CAD build for the part. Positions are in the model's coordinates, mm. A direction names the side the tool comes from. Round coordinates to 2 decimals unless told otherwise and drop trailing zeros. Loops run counter-clockwise (first coordinate to the right, second up) from the corner with the lowest first, then second, coordinate; pieces in that order, holes last. Notation, with made-up numbers: (-20, -25) - (-16, -25) arc R34 cw to (-16, 7) - close; hole circle Ø9 at (24, -28). An arc over 180 degrees is marked (long way). Use one line per item in the form item = value.
from build123d import *

# Parameters (mm, degrees)
SKETCH_1_W          = 25.2
SKETCH_1_H          = 20
EXTRUDE_1_DEPTH     = 2
SKETCH_2_W          = 2.5
SKETCH_2_H          = 20
EXTRUDE_2_DEPTH     = 20
SKETCH_3_R          = 1.5
CUT_EXTRUDE_1_DEPTH = 34.690354703
SKETCH_4_R          = 8.5
EXTRUDE_3_DEPTH     = 3
SKETCH_5_R          = 7.5
EXTRUDE_4_DEPTH     = 8
SKETCH_6_R          = 7
EXTRUDE_5_DEPTH     = 18
SKETCH_10_R         = 9.319748931
SKETCH_10_W         = 12
SKETCH_10_H         = 12
CUT_EXTRUDE_4_DEPTH = 15
FILLET_2_R          = 1.5
SKETCH_12_R         = 7.5
CUT_EXTRUDE_5_DEPTH = 26
SKETCH_13_W         = 0.35
SKETCH_13_H         = 1.1


with BuildPart() as part:
    # 草图1 → 凸台-拉伸1 (new body)
    with BuildSketch(Plane(origin=(0, 0, 0), x_dir=(1, 0, 0), z_dir=(0, 1, 0))):
        Rectangle(SKETCH_1_W, SKETCH_1_H)
    extrude(amount=EXTRUDE_1_DEPTH)

    # 草图2 → 凸台-拉伸2 (add)
    with BuildSketch(Plane.XZ):
        with Locations((-11.35, 0)):
            Rectangle(SKETCH_2_W, SKETCH_2_H)
        with Locations((11.35, 0)):
            Rectangle(SKETCH_2_W, SKETCH_2_H)
    extrude(amount=EXTRUDE_2_DEPTH)

    # 草图3 → 切除-拉伸1 (cut, through all)
    with BuildSketch(Plane(origin=(12.6, 0, 0), x_dir=(0, 0, -1), z_dir=(1, 0, 0))):
        with Locations((-4, -17)):
            Circle(SKETCH_3_R)
        with Locations((4, -17)):
            Circle(SKETCH_3_R)
        with Locations((4, -3)):
            Circle(SKETCH_3_R)
        with Locations((-4, -3)):
            Circle(SKETCH_3_R)
    extrude(amount=-CUT_EXTRUDE_1_DEPTH, mode=Mode.SUBTRACT)

    # 草图4 → 凸台-拉伸3 (add)
    with BuildSketch(Plane(origin=(0, 2, 0), x_dir=(1, 0, 0), z_dir=(0, 1, 0))):
        with Locations(Location((0, 0, 0), (0, 0, 270))):
            Circle(SKETCH_4_R)
    extrude(amount=EXTRUDE_3_DEPTH)

    # 草图5 → 凸台-拉伸4 (add)
    with BuildSketch(Plane(origin=(0, 5, 0), x_dir=(1, 0, 0), z_dir=(0, 1, 0))):
        with Locations(Location((0, 0, 0), (0, 0, 270))):
            Circle(SKETCH_5_R)
    extrude(amount=EXTRUDE_4_DEPTH)

    # 草图6 → 凸台-拉伸5 (add)
    with BuildSketch(Plane(origin=(0, 13, 0), x_dir=(1, 0, 0), z_dir=(0, 1, 0))):
        with Locations(Location((0, 0, 0), (0, 0, 270))):
            Circle(SKETCH_6_R)
    extrude(amount=EXTRUDE_5_DEPTH)

    # 草图10 → 切除-拉伸4 (cut)
    with BuildSketch(Plane(origin=(0, 31, 0), x_dir=(1, 0, 0), z_dir=(0, 1, 0))):
        Circle(SKETCH_10_R)
        Rectangle(SKETCH_10_W, SKETCH_10_H, mode=Mode.SUBTRACT)
    extrude(amount=-CUT_EXTRUDE_4_DEPTH, mode=Mode.SUBTRACT)

    # 圆角2
    fillet_2_edges = [part.edges().sort_by_distance(p)[0] for p in [
        (0, 2, -8.5),
    ]]
    fillet(fillet_2_edges, radius=FILLET_2_R - 0.0001)  # a hair under: the kernel refuses the full size

    # 草图12 → 切除-拉伸5 (cut)
    with BuildSketch(Plane(origin=(0, 13, 0), x_dir=(1, 0, 0), z_dir=(0, 1, 0))):
        with Locations(Location((0, 0, 0), (0, 0, 270))):
            Circle(SKETCH_12_R)
    extrude(amount=CUT_EXTRUDE_5_DEPTH, mode=Mode.SUBTRACT)

    # 草图13 → 切除-旋转1 (revolve, cut)
    with BuildSketch(Plane(origin=(0, 0, 0), x_dir=(0, 0, -1), z_dir=(1, 0, 0)), mode=Mode.PRIVATE) as cut_revolve_1_sk:
        with Locations((7.325, 10.55)):
            Rectangle(SKETCH_13_W, SKETCH_13_H)
    revolve(cut_revolve_1_sk.sketch.rotate(Axis((0, 13, 0), (0, -1, 0)), 180), axis=Axis((0, 13, 0), (0, -1, 0)), mode=Mode.SUBTRACT)


solid = part.part
1) Slice it at A-A (y = -8). Write the cut outline in (x, z), plus the area to 3 significant figures.
Report:
outline = (-12.6, -10) - (-10.1, -10) - (-10.1, 10) - (-12.6, 10) - close; (10.1, -10) - (12.6, -10) - (12.6, 10) - (10.1, 10) - close
area = 100 mm^2
2) Tool access for faces 5 (the cylindrical face through (11.37, -2.55, -5.43)), 6 (the cylindrical face through (0.33, 12.037, -7.493)): list every direction of +Z, -Z, +X, -X, +Y, -Y with a clear straight run to the whole face (end or side of a thin tool).
Report:
face_5 = +X, -X
face_6 = +Y
3) Slice it at B-B (y = -17.5). Write the cut outline in (x, z), plus the area to 3 significant figures.
Report:
outline = (-12.6, -10) - (-10.1, -10) - (-10.1, -5.41) - (-12.6, -5.41) - close; (-12.6, -2.59) - (-10.1, -2.59) - (-10.1, 2.59) - (-12.6, 2.59) - close; (-12.6, 5.41) - (-10.1, 5.41) - (-10.1, 10) - (-12.6, 10) - close; (10.1, -10) - (12.6, -10) - (12.6, -5.41) - (10.1, -5.41) - close; (10.1, -2.59) - (12.6, -2.59) - (12.6, 2.59) - (10.1, 2.59) - close; (10.1, 5.41) - (12.6, 5.41) - (12.6, 10) - (10.1, 10) - close
area = 71.7 mm^2
4) Slice it at D-D (z = -4). State how many separate pieces and enclosed holes the cut face has, plus the area to 3 significant figures.
Report:
separate_pieces = 5
enclosed_holes = 0
area = 267 mm^2
5) Drill centre lines: probe 1 along Y at (x, z) = (10.8, -4); probe 2 along X at (y, z) = (-17.5, 7.25); probe 3 along Y at (x, z) = (10.75, 9). Where is each one in solid material? Low to high.
Report:
probe_1 = -20 to -18.5, -15.5 to -4.5, -1.5 to 2
probe_2 = -12.6 to -10.1, 10.1 to 12.6
probe_3 = -20 to 2
6) Flat gauge pins, fed straight in: pin 1 (6 mm diameter, centred on x = 0, z = -2, fed in from -Y); pin 2 (5 mm diameter, centred on y = 5.5, z = 8, fed in from +X); pin 3 (6 mm diameter, centred on x = -9.5, y = 9, fed in from +Z); pin 4 (12 mm diameter, centred on y = 6, z = -2, fed in from -X). Where does each tip first touch, or does it go through?
Report:
pin_1 = 0
pin_2 = 6.44
pin_3 = 3.74
pin_4 = -12.6
7) Two-plate mould, pull along X, no slides. Class faces 1 (the cylindrical face through (8.428, 4.239, -1.107)), 2 (the flat face through (0, 13, 0)), 3 (the flat face through (0, 0, 0)), 4 (the flat face through (-10.1, -10, 0)): +X half, -X half, draft (parallel to the pull), parting line (faces both ways), or undercut.
Report:
face_1 = parting line
face_2 = draft
face_3 = undercut
face_4 = undercut
